Check sheet for the modelled part. Datum: model origin and axes. Units: mm. Face numbers are marked on the shaded views. A direction names the side the tool comes from. Coordinates: 2 decimals unless noted, no trailing zeros. Order: outer loops, then holes, each group sorted by start corner. A loop starts at its lowest first (then second) coordinate and runs counter-clockwise, first axis right, second up.
1. Cross-section at C-C (x = 1.75). Enter the section's corners in (y, z).
2. Thickness scan on line 1 (X direction, y = 13, z = 4); line 2 (Y direction, x = 13.25, z = 5.5). Record the ranges inside material, lowest first.
3. Set-up check for the marked faces 1 and 2: record each of +Z, -Z, +X, -X, +Y, -Y from which the full face is reachable in a straight line by a thin tool's end or side.
4. Gauge pin test, flat ends, axial feed: pin 1 Ø23 at (y, z) = (48.46, 22) entering from +X; pin 2 Ø5 at (x, z) = (7.37, 6.19) entering from +Y; pin 3 Ø4 at (y, z) = (64.3, 37.63) entering from -X. Record the tip position at first contact, or that the pin passes through.
5. Cross-section at D-D (z = 30). Enter the section's corners in (x, y).
6. Cross-section at B-B (y = 32). Enter the section's corners in (x, z).
7. Cross-section at A-A (z = 22). Enter the section's corners in (x, y).
```python
from build123d import *

# Parameters (mm, degrees)
EXTRUDE_THIN1_DEPTH = 44
SKETCH2_R           = 19
CUT_EXTRUDE1_DEPTH  = 85.310438262
SKETCH3_R           = 2
CUT_EXTRUDE2_DEPTH  = 85.310438262
SKETCH4_R           = 1.5
CUT_EXTRUDE3_DEPTH  = 85.310438262


with BuildPart() as part:
    # Sketch1 → Extrude-Thin1 (new body)
    with BuildSketch(Plane.XY):
        Polygon((0, 0), (15, 0), (15, 70), (16.5, 70), (16.5, -1.5), (0, -1.5), align=None)
    extrude(amount=EXTRUDE_THIN1_DEPTH)

    # Sketch2 → Cut-Extrude1 (cut, through all)
    with BuildSketch(Plane(origin=(16.5, 0, 0), x_dir=(0, 0, -1), z_dir=(1, 0, 0))):
        with Locations((-22, 48.459332075)):
            Circle(SKETCH2_R)
    extrude(amount=-CUT_EXTRUDE1_DEPTH, mode=Mode.SUBTRACT)

    # Sketch3 → Cut-Extrude2 (cut, through all)
    with BuildSketch(Plane(origin=(0, 0, 0), x_dir=(1, 0, 0), z_dir=(0, 1, 0))):
        with Locations(Location((7.370084174, -6.191389664, 0), (0, 0, 270))):
            Circle(SKETCH3_R)
        with Locations(Location((7.370084174, -37.808610336, 0), (0, 0, 270))):
            Circle(SKETCH3_R)
    extrude(amount=-CUT_EXTRUDE2_DEPTH, mode=Mode.SUBTRACT)

    # Sketch4 → Cut-Extrude3 (cut, through all)
    with BuildSketch(Plane(origin=(16.5, 0, 0), x_dir=(0, 0, -1), z_dir=(1, 0, 0))):
        with Locations((-37.627392524, 64.304718843)):
            Circle(SKETCH4_R)
        with Locations((-6.044034896, 64.304718843)):
            Circle(SKETCH4_R)
        with Locations((-37.627392524, 32.719245679)):
            Circle(SKETCH4_R)
        with Locations((-6.044034896, 32.719245679)):
            Circle(SKETCH4_R)
    extrude(amount=-CUT_EXTRUDE3_DEPTH, mode=Mode.SUBTRACT)


solid = part.part
```
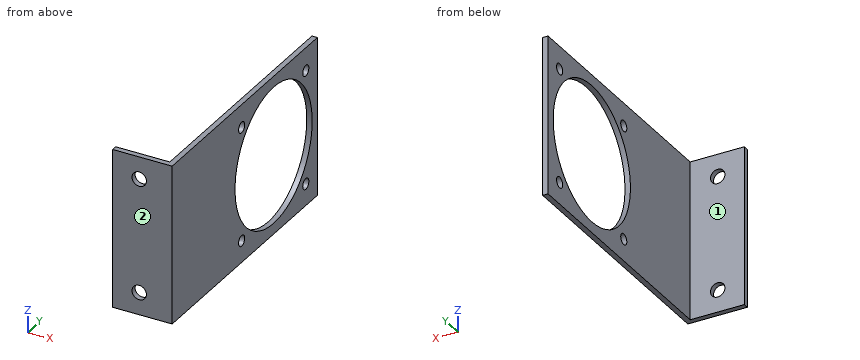
Data:
1. outline: (-1.5, 0) - (0, 0) - (0, 44) - (-1.5, 44) - close
2. line 1: x = 15 to 16.5
2. line 2: y = -1.5 to 0
3. face 1: +Z, -Z, -X, +Y
3. face 2: +Z, -Z, +X, -X, -Y
4. pin 1: passes through
4. pin 2: stops at y = 0
4. pin 3: stops at x = 15
5. outline: (0, -1.5) - (16.5, -1.5) - (16.5, 31.23) - (15, 31.23) - (15, 0) - (0, 0) - close; (15, 65.69) - (16.5, 65.69) - (16.5, 70) - (15, 70) - close
6. outline: (15, 0) - (16.5, 0) - (16.5, 4.73) - (15, 4.73) - close; (15, 7.36) - (16.5, 7.36) - (16.5, 12.51) - (15, 12.51) - close; (15, 31.49) - (16.5, 31.49) - (16.5, 36.31) - (15, 36.31) - close; (15, 38.94) - (16.5, 38.94) - (16.5, 44) - (15, 44) - close
7. outline: (0, -1.5) - (16.5, -1.5) - (16.5, 29.46) - (15, 29.46) - (15, 0) - (0, 0) - close; (15, 67.46) - (16.5, 67.46) - (16.5, 70) - (15, 70) - close
